Geometry check sheet. Reference: the model listing, model coordinates, mm. A direction names the side the tool comes from. Give positions to 0.01 mm unless a question says otherwise; leave off trailing zeros. Order: outer loops, then holes, each group sorted by start corner. A loop starts at its lowest first (then second) coordinate and runs counter-clockwise, first axis right, second up. Notation, with made-up numbers: M 84.25,85.5 L 137.25,85.5 A26 cw 137.25,112.5 Z; hole C 85,-19 d9. An arc over 180 degrees is marked long. Answer as a JSON object with one key per item and string values. Group by question number.
from build123d import *

# Parameters (mm, degrees)
BOSS_EXTRUDE1_DEPTH            = 40
SKETCH2_W                      = 40
SKETCH2_H                      = 30
BOSS_EXTRUDE2_DEPTH            = 20
BOSS_EXTRUDE3_DEPTH            = 30
CUT_EXTRUDE1_DEPTH             = 30
SKETCH5_W                      = 70
SKETCH5_H                      = 40
BOSS_EXTRUDE4_DEPTH            = 10
SKETCH6_W                      = 20
SKETCH6_H                      = 20
CUT_EXTRUDE2_DEPTH             = 41
F_10_0_10_DIAMETER_HOLE1_D     = 10
F_10_0_10_DIAMETER_HOLE1_DEPTH = 40
FILLET1_R                      = 20


with BuildPart() as part:
    # Sketch1 → Boss-Extrude1 (new body)
    with BuildSketch(Plane(origin=(0, 0, 0), x_dir=(0, -1, 0), z_dir=(-1, 0, 0))):
        Polygon((-10, -16), (-40, -20), (-10, -20), align=None)
    extrude(amount=-BOSS_EXTRUDE1_DEPTH)

    # Sketch2 → Boss-Extrude2 (add)
    with BuildSketch(Plane(origin=(0, 0, -20), x_dir=(-1, 0, 0), z_dir=(0, 0, -1))):
        with Locations((-20, 25)):
            Rectangle(SKETCH2_W, SKETCH2_H)
    extrude(amount=BOSS_EXTRUDE2_DEPTH)

    # Sketch3 → Boss-Extrude3 (add)
    with BuildSketch(Plane(origin=(40, 0, 0), x_dir=(0, 0, -1), z_dir=(1, 0, 0))):
        Polygon((40, 10), (0, 10), (20, 40), (40, 40), align=None)
    extrude(amount=BOSS_EXTRUDE3_DEPTH)

    # Sketch4 → Cut-Extrude1 (cut)
    with BuildSketch(Plane(origin=(70, 0, 0), x_dir=(0, 0, -1), z_dir=(1, 0, 0))):
        Polygon((20, 40), (0, 10), (30, 10), (30, 30), (40, 30), (40, 40), align=None)
    extrude(amount=-CUT_EXTRUDE1_DEPTH, mode=Mode.SUBTRACT)

    # Sketch5 → Boss-Extrude4 (add)
    with BuildSketch(Plane.XZ.offset(-10)):
        with Locations((35, -20)):
            Rectangle(SKETCH5_W, SKETCH5_H)
    extrude(amount=BOSS_EXTRUDE4_DEPTH)

    # Sketch6 → Cut-Extrude2 (cut, through all)
    with BuildSketch(Plane(origin=(0, 0, -40), x_dir=(-1, 0, 0), z_dir=(0, 0, -1))):
        with Locations((-20, 30)):
            Rectangle(SKETCH6_W, SKETCH6_H)
    extrude(amount=-CUT_EXTRUDE2_DEPTH, mode=Mode.SUBTRACT)

    # Ø10.0 (10) Diameter Hole1
    with Locations(Plane(origin=(0, 0, 0), x_dir=(-1, 0, 0), z_dir=(0, -1, 0))):
        with Locations((-55, 15)):
            Hole(F_10_0_10_DIAMETER_HOLE1_D / 2, depth=F_10_0_10_DIAMETER_HOLE1_DEPTH)

    # Fillet1
    fillet1_edges = [part.edges().sort_by_distance(p)[0] for p in [
        (70, 30, -35),
    ]]
    fillet(fillet1_edges, radius=FILLET1_R)


solid = part.part
1. Cross-section at A-A (z = -15). Record the cut outline in (x, y).
2. Access from +Z, -Z, +X, -X, +Y, -Y to the whole of each face (thin tool, end or side, straight path). Record for faces 1 (the flat face through (19.72, 18.123, -17.083)), 2 (the flat face through (52, 20, -30)), 3 (the flat face through (10, 30, -29)), 4 (the flat face through (45, 30, -35)).
3. Release check for a two-part mould opening along X. For faces 5 (the flat face through (42, 10, -11)), 6 (the flat face through (30, 30, -29)), 7 (the flat face through (70, 5, -20)) record: released by +X, released by -X, zero draft, split by the parting line, or undercut.
4. Thickness scan on line 1 along Z through (x, y) = (55, 8); line 2 along X through (y, z) = (25, -24); line 3 along Z through (x, y) = (46.5, 22.5). Record the ranges inside material, lowest first. Write a range as [from, to].
5. Depth check by flat-ended pin: pin 1 (6 mm diameter, centred on x = 57.5, y = 22, fed in from +Z); pin 2 (5 mm diameter, centred on x = 45, z = -36, fed in from +Y); pin 3 (6 mm diameter, centred on y = 32.5, z = -28, fed in from +X). Enter the tip coordinate at first touch or a pass-through.
6. Cross-section at C-C (z = -21). Record the cut outline in (x, y).
7. Cross-section at D-D (x = 45). Record the cut outline in (y, z).
8. Cross-section at B-B (y = 22.5). Record the cut outline in (x, z).
Report:
{
 "1": {"outline": "M 0,0 L 50,0 L 50,10 L 0,10 Z; M 60,0 L 70,0 L 70,10 L 60,10 Z"},
 "2": {"face 1": "+Z, +X, -X, +Y", "face 2": "+Z, +X, +Y", "face 3": "+Z, -Z, +Y", "face 4": "+Z, -Z, +X, +Y"},
 "3": {"face 5": "zero draft", "face 6": "undercut", "face 7": "released by +X"},
 "4": {"line 1": "z = [-40, -20], [-10, 0]", "line 2": "x = [0, 10], [30, 40]", "line 3": "z = [-40, -30]"},
 "5": {"pin 1": "stops at z = -30", "pin 2": "stops at y = 30", "pin 3": "stops at x = 40"},
 "6": {"outline": "M 0,0 L 70,0 L 70,10 L 40,10 L 40,40 L 30,40 L 30,20 L 10,20 L 10,40 L 0,40 Z"},
 "7": {"outline": "M 0,-40 L 30,-40 L 30,-30 L 10,-30 L 10,0 L 0,0 Z"},
 "8": {"outline": "M 0,-40 L 10,-40 L 10,-17.67 L 0,-17.67 Z; M 30,-40 L 65.61,-40 L 65.61,-30 L 40,-30 L 40,-17.67 L 30,-17.67 Z"}
}
